```python
from build123d import *

# Parameters (mm, degrees)
BOSS_EXTRUDE2_DEPTH      = 200
CUT_EXTRUDE10_DEPTH      = 138.5000001
CUT_EXTRUDE10_DEPTH_BACK = 138.5000001


with BuildPart() as part:
    # Sketch18 → Boss-Extrude2 (new body)
    with BuildSketch(Plane.XY):
        with BuildLine():
            Line((137.5, 90.870921856), (137.5, 15.1))
            Line((137.5, 15.1), (-137.5, 15.1))
            Line((-137.5, 15.1), (-137.5, 90.870921856))
            add(Edge.make_bspline(
                [(137.5, 90.870921856), (0, 133.155906783), (-137.5, 90.870921856)],
                knots=[4.113742813, 4.113742813, 4.113742813, 5.311035148, 5.311035148, 5.311035148], degree=2, weights=[1, 0.82609929, 1]))
        make_face()
    extrude(amount=-BOSS_EXTRUDE2_DEPTH)

    # Sketch15 → Cut-Extrude10 (cut, two sides)
    with BuildSketch(Plane(origin=(0, 0, 0), x_dir=(0, 0, -1), z_dir=(1, 0, 0))) as cut_extrude10_sk:
        Polygon((0, 110), (0, 95), (200, -5), (200, 110), align=None)
    extrude(amount=CUT_EXTRUDE10_DEPTH, mode=Mode.SUBTRACT)
    extrude(cut_extrude10_sk.sketch, amount=-CUT_EXTRUDE10_DEPTH_BACK, mode=Mode.SUBTRACT)


solid = part.part
```
The listing builds one solid part. Answer for the finished solid, in the listing's coordinates (mm). Coordinates: 2 decimals unless noted, no trailing zeros. Loops run counter-clockwise (first coordinate to the right, second up) from the corner with the lowest first, then second, coordinate; pieces in that order, holes last. Notation, with made-up numbers: (77, -1.75) -> (123, -1.75) arc R20 ccw to (123, 27.25) -> close; hole circle Ø4 at (-13.5, 46). An arc over 180 degrees is marked (long way). Return JSON: item names as keys, results as strings. Group by question number.
(1) A cutting plane is placed at A-A on y = 43. Write down the section's boundary in (x, z).
(2) Given pin 1 Ø1 at (x, y) = (5.5, 37.5) entering from -Z; pin 2 Ø8 at (x, z) = (-71, -117.5) entering from +Y; pin 3 Ø1.5 at (x, y) = (76.5, 42.5) entering from -Z, each flat-ended and moving along its own axis, determine where each tip first touches the part or whether it passes through.
(3) A cutting plane is placed at C-C on x = -86. Write down the section's boundary in (y, z), and give its area (3 significant figures).
(4) Find the intervals of material crossed by probe 1 along Y at (x, z) = (-104, -72); probe 2 along Z at (x, y) = (-106.5, 47); probe 3 along Z at (x, y) = (84.5, 56), in increasing order. Write a range as from..to.
(5) A cutting plane is placed at B-B on z = -142. Write down the section's boundary in (x, y), and give its area (3 significant figures).
The answers:
{
 "1": {"outline": "(-137.5, -104) -> (137.5, -104) -> (137.5, 0) -> (-137.5, 0) -> close"},
 "2": {"pin 1": "stops at z = -116", "pin 2": "stops at y = 38.25", "pin 3": "stops at z = -106.5"},
 "3": {"outline": "(15.1, -159.8) -> (95, 0) -> (15.1, 0) -> close", "area": "6,380 mm^2"},
 "4": {"probe 1": "y = 15.1..59", "probe 2": "z = -96..0", "probe 3": "z = -78..0"},
 "5": {"outline": "(-137.5, 15.1) -> (137.5, 15.1) -> (137.5, 24) -> (-137.5, 24) -> close", "area": "2,450 mm^2"}
}
